```python
from build123d import *

# Parameters (mm, degrees)
SKETCH1_W           = 15
SKETCH1_H           = 45
BOSS_EXTRUDE1_DEPTH = 2.2
SKETCH1_3_W         = 20
SKETCH1_3_H         = 50
SKETCH1_3_W_2       = 15
SKETCH1_3_H_2       = 45
BOSS_EXTRUDE2_DEPTH = 2.5
SKETCH1_4_W         = 20
SKETCH1_4_H         = 50
SKETCH1_4_R         = 4.1
BOSS_EXTRUDE3_DEPTH = 2.5
FILLET1_R           = 2
SKETCH1_5_R         = 3.1
BOSS_EXTRUDE4_DEPTH = 2.5
FILLET2_R           = 10
CUT_EXTRUDE2_DEPTH  = 4
SKETCH3_OUTSIDE_W   = 41.892
SKETCH3_OUTSIDE_H   = 119.192
CUT_EXTRUDE3_DEPTH  = 74.159346635


with BuildPart() as part:
    # Sketch1 → Boss-Extrude1 (new body)
    with BuildSketch(Plane(origin=(0, 0, 0), x_dir=(1, 0, 0), z_dir=(0, 1, 0))):
        Rectangle(SKETCH1_W, SKETCH1_H)
        with BuildLine():
            ThreePointArc((-3.894544437, -4.023993492), (-5.599998379, 0.004260474), (-3.88841703, 4.029914763))
            Line((-3.88841703, 4.029914763), (-3.88841703, 8.505312122))
            ThreePointArc((-3.88841703, 8.505312122), (-3.870707724, 8.925763598), (-3.817705253, 9.343236712))
            Line((-3.817705253, 9.343236712), (-2.664584371, 16.126741161))
            ThreePointArc((-2.664584371, 16.126741161), (-2.610617779, 16.555799687), (-2.593926654, 16.987916591))
            ThreePointArc((-2.593926654, 16.987916591), (0, 19.6), (2.606045235, 17.000007028))
            ThreePointArc((2.606045235, 17.000007028), (2.623754541, 16.579555552), (2.676757012, 16.162082438))
            Line((2.676757012, 16.162082438), (3.829877895, 9.378577989))
            ThreePointArc((3.829877895, 9.378577989), (3.882880366, 8.961104875), (3.900589672, 8.540653399))
            Line((3.900589672, 8.540653399), (3.900589672, 4.018133922))
            ThreePointArc((3.900589672, 4.018133922), (5.157678846, 2.181364004), (5.6, 0))
            ThreePointArc((5.6, 0), (5.156037667, -2.185240393), (3.894544437, -4.023993492))
            Line((3.894544437, -4.023993492), (3.894544437, -8.540646372))
            ThreePointArc((3.894544437, -8.540646372), (3.876835131, -8.961097847), (3.82383266, -9.378570962))
            Line((3.82383266, -9.378570962), (2.670711777, -16.16207541))
            ThreePointArc((2.670711777, -16.16207541), (2.617709306, -16.579548524), (2.6, -17))
            ThreePointArc((2.6, -17), (0, -19.6), (-2.6, -17))
            ThreePointArc((-2.6, -17), (-2.617709306, -16.579548524), (-2.670711777, -16.16207541))
            Line((-2.670711777, -16.16207541), (-3.82383266, -9.378570962))
            ThreePointArc((-3.82383266, -9.378570962), (-3.876835131, -8.961097847), (-3.894544437, -8.540646372))
            Line((-3.894544437, -8.540646372), (-3.894544437, -4.023993492))
        make_face(mode=Mode.SUBTRACT)
    extrude(amount=-BOSS_EXTRUDE1_DEPTH)

    # Sketch1<3> → Boss-Extrude2 (add)
    # profile 1 of 2: a face of its own
    with BuildSketch(Plane(origin=(0, 0, 0), x_dir=(1, 0, 0), z_dir=(0, 1, 0))):
        Rectangle(SKETCH1_3_W, SKETCH1_3_H)
        Rectangle(SKETCH1_3_W_2, SKETCH1_3_H_2, mode=Mode.SUBTRACT)
    # profile 2 of 2: a face of its own
    with BuildSketch(Plane(origin=(0, 0, 0), x_dir=(1, 0, 0), z_dir=(0, 1, 0))):
        Rectangle(SKETCH1_3_W_2, SKETCH1_3_H_2)
        with BuildLine():
            ThreePointArc((-3.894544437, -4.023993492), (-5.599998379, 0.004260474), (-3.88841703, 4.029914763))
            Line((-3.88841703, 4.029914763), (-3.88841703, 8.505312122))
            ThreePointArc((-3.88841703, 8.505312122), (-3.870707724, 8.925763598), (-3.817705253, 9.343236712))
            Line((-3.817705253, 9.343236712), (-2.664584371, 16.126741161))
            ThreePointArc((-2.664584371, 16.126741161), (-2.610617779, 16.555799687), (-2.593926654, 16.987916591))
            ThreePointArc((-2.593926654, 16.987916591), (0, 19.6), (2.606045235, 17.000007028))
            ThreePointArc((2.606045235, 17.000007028), (2.623754541, 16.579555552), (2.676757012, 16.162082438))
            Line((2.676757012, 16.162082438), (3.829877895, 9.378577989))
            ThreePointArc((3.829877895, 9.378577989), (3.882880366, 8.961104875), (3.900589672, 8.540653399))
            Line((3.900589672, 8.540653399), (3.900589672, 4.018133922))
            ThreePointArc((3.900589672, 4.018133922), (5.157678846, 2.181364004), (5.6, 0))
            ThreePointArc((5.6, 0), (5.156037667, -2.185240393), (3.894544437, -4.023993492))
            Line((3.894544437, -4.023993492), (3.894544437, -8.540646372))
            ThreePointArc((3.894544437, -8.540646372), (3.876835131, -8.961097847), (3.82383266, -9.378570962))
            Line((3.82383266, -9.378570962), (2.670711777, -16.16207541))
            ThreePointArc((2.670711777, -16.16207541), (2.617709306, -16.579548524), (2.6, -17))
            ThreePointArc((2.6, -17), (0, -19.6), (-2.6, -17))
            ThreePointArc((-2.6, -17), (-2.617709306, -16.579548524), (-2.670711777, -16.16207541))
            Line((-2.670711777, -16.16207541), (-3.82383266, -9.378570962))
            ThreePointArc((-3.82383266, -9.378570962), (-3.876835131, -8.961097847), (-3.894544437, -8.540646372))
            Line((-3.894544437, -8.540646372), (-3.894544437, -4.023993492))
        make_face(mode=Mode.SUBTRACT)
    extrude(amount=-BOSS_EXTRUDE2_DEPTH)

    # Sketch1<4> → Boss-Extrude3 (add)
    with BuildSketch(Plane(origin=(0, 0, 0), x_dir=(1, 0, 0), z_dir=(0, 1, 0))):
        Rectangle(SKETCH1_4_W, SKETCH1_4_H)
        with Locations(Location((0, 0, 0), (0, 0, 270))):
            Circle(SKETCH1_4_R, mode=Mode.SUBTRACT)
    extrude(amount=BOSS_EXTRUDE3_DEPTH)

    # Fillet1
    fillet1_edges = [part.edges().sort_by_distance(p)[0] for p in [
        (-3.88841703, -1.25, -4.029914763),
        (-3.894544437, -1.25, 4.023993492),
        (3.894544437, -1.25, 4.023993492),
        (3.900589672, -1.25, -4.018133922),
    ]]
    fillet(fillet1_edges, radius=FILLET1_R)

    # Sketch1<5> → Boss-Extrude4 (add, symmetric)
    with BuildSketch(Plane(origin=(0, 0, 0), x_dir=(1, 0, 0), z_dir=(0, 1, 0))):
        with BuildLine():
            ThreePointArc((-10, 62.3), (0, 72.3), (10, 62.3))
            Line((10, 62.3), (10, 25))
            Line((10, 25), (-10, 25))
            Line((-10, 25), (-10, 62.3))
        make_face()
        with Locations(Location((0, 62.3, 0), (0, 0, 270))):
            Circle(SKETCH1_5_R, mode=Mode.SUBTRACT)
    extrude(amount=BOSS_EXTRUDE4_DEPTH, both=True)

    # Fillet2
    fillet2_edges = [part.edges().sort_by_distance(p)[0] for p in [
        (10, 0, 25),
        (-10, 0, 25),
    ]]
    fillet(fillet2_edges, radius=FILLET2_R - 0.0001)  # a hair under: the kernel refuses the full size

    # Sketch2 → Cut-Extrude2 (cut)
    # profile 1 of 4: a face of its own
    with BuildSketch(Plane.XZ.offset(2.5)):
        Polygon((5.973502692, -40.744870683), (-2.986751346, -35.571665602), (-2.986751346, -45.918075763), align=None)
        Polygon((5.773502692, -40.744870683), (-2.886751346, -35.744870683), (-2.886751346, -45.744870683), align=None, mode=Mode.SUBTRACT)
    # profile 2 of 4: a face of its own
    with BuildSketch(Plane.XZ.offset(2.5)):
        Polygon((5.973502692, -24.744870683), (-2.986751346, -19.571665602), (-2.986751346, -29.918075763), align=None)
        Polygon((5.773502692, -24.744870683), (-2.886751346, -19.744870683), (-2.886751346, -29.744870683), align=None, mode=Mode.SUBTRACT)
    # profile 3 of 4: a face of its own
    with BuildSketch(Plane.XZ.offset(2.5)):
        Polygon((-3.086751346, -48.744870683), (5.873502692, -43.571665602), (5.873502692, -53.918075763), align=None)
        Polygon((5.773502692, -53.744870683), (-2.886751346, -48.744870683), (5.773502692, -43.744870683), align=None, mode=Mode.SUBTRACT)
    # profile 4 of 4: a face of its own
    with BuildSketch(Plane.XZ.offset(2.5)):
        Polygon((-3.086751346, -32.744870683), (5.873502692, -27.571665602), (5.873502692, -37.918075763), align=None)
        Polygon((5.773502692, -37.744870683), (-2.886751346, -32.744870683), (5.773502692, -27.744870683), align=None, mode=Mode.SUBTRACT)
    extrude(amount=-CUT_EXTRUDE2_DEPTH, mode=Mode.SUBTRACT)

    # Sketch3 outside → Cut-Extrude3 (cut, through all)
    with BuildSketch(Plane.XZ.offset(2.5)):
        with Locations((0, -23.65)):
            Rectangle(SKETCH3_OUTSIDE_W, SKETCH3_OUTSIDE_H)
        with BuildLine():
            Line((10, -51.256214284), (10, 15))
            ThreePointArc((10, 15), (7.071067812, 22.071067812), (0, 25))
            ThreePointArc((0, 25), (-7.071067812, 22.071067812), (-10, 15))
            Line((-10, 15), (-10, -52.147572729))
            add(Edge.make_bspline(
                [(10, -51.256214284), (9.785135746, -51.909968828), (9.078957117, -53.953043182), (7.795150781, -57.091457155), (6.013003778, -60.33910848), (4.122796637, -62.728314915), (2.078800951, -64.258582197), (-0.15, -64.79554013), (-2.378800951, -64.258582197), (-4.422796637, -62.728314915), (-6.313003778, -60.33910848), (-8.095150781, -57.091457155), (-9.260115035, -54.243566479), (-9.877905488, -52.501784004), (-10, -52.147572729)],
                knots=[0.471097659, 0.471097659, 0.471097659, 0.471097659, 0.474472001, 0.481696232, 0.487703698, 0.492583405, 0.496543603, 0.5, 0.503456397, 0.507416595, 0.512296302, 0.518303768, 0.525527999, 0.527365119, 0.527365119, 0.527365119, 0.527365119], degree=3))
        make_face(mode=Mode.SUBTRACT)
    extrude(amount=-CUT_EXTRUDE3_DEPTH, mode=Mode.SUBTRACT)


solid = part.part
```
Could you check a few things on this model? Use its own coordinates, in mm. A direction names the side the tool comes from. Coordinates: 2 decimals unless noted, no trailing zeros. Order: outer loops, then holes, each group sorted by start corner. A loop starts at its lowest first (then second) coordinate and runs counter-clockwise, first axis right, second up. Notation, with made-up numbers: M 31,62.5 L 51,62.5 A25 cw 51,88.5 Z; hole C 37,-39.5 d5. An arc over 180 degrees is marked long. Use one line per item in the form item = value. Start each with the question number.
1. Suppose I cut it at C-C on z = 12.5. Write out the boundary of the cut face in (x, y).
2. On a 3-axis mill with a long thin cutter (end or side, diameter ignored), from which of +Z, -Z, +X, -X, +Y, -Y can I reach the whole of each face in a straight line? I mean faces 4 (the flat face through (1, -2.5, -41)), 5 (the cylindrical face through (5.6, -1.2, 0)). Say none if no direction works.
3. We'd pull the mould along Z, two halves only. Please class faces 1 (the flat face through (0, -2.5, -20)), 2 (the cylindrical face through (7.15, -0.04, 21.99)), 3 (the flat face through (3.901, -1, -7)): +Z half, -Z half, draft (parallel to the pull), parting line (faces both ways), or undercut.
4. For pin 1 (2 mm diameter, centred on x = -7.5, y = -1, fed in from -Z); pin 2 (2 mm diameter, centred on x = 0.5, y = 1, fed in from -Z), each with a flat end and sliding along its axis, tell me the tip position at first contact or that it passes through.
5. Suppose I cut it at A-A on z = 0. Write out the boundary of the cut face in (x, y), then the cut area to 3 significant figures.
6. Suppose I cut it at D-D on z = -29. Write out the boundary of the cut face in (x, y).
7. Suppose I cut it at B-B on y = -1.15. Count the separate pieces of the cut face and the enclosed holes in it, then the cut area to 3 significant figures.
8. Please list where these lines run through material, in increasing order: line 1 (X direction, y = -0.2, z = -7.5); line 2 (X direction, y = 1.35, z = 0); line 3 (Z direction, x = -1.5, y = 2.05).
Geometry says:
q1.outline = M -10,-2.5 L -3.29,-2.5 L -3.29,0 L 3.29,0 L 3.29,-2.5 L 10,-2.5 L 10,2.5 L -10,2.5 Z
q2.face_4 = +Z, -Z, +X, -X, -Y
q2.face_5 = -Y
q3.face_1 = draft
q3.face_2 = +Z half
q3.face_3 = undercut
q4.pin_1 = -59.88
q4.pin_2 = -59.59
q5.outline = M -10,-2.5 L -5.6,-2.5 L -5.6,0 L -4.1,0 L -4.1,2.5 L -10,2.5 Z; M 4.1,0 L 5.6,0 L 5.6,-2.5 L 10,-2.5 L 10,2.5 L 4.1,2.5 Z
q5.area = 51.5 mm^2
q6.outline = M -10,-2.5 L -2.99,-2.5 L -2.99,1.5 L -2.89,1.5 L -2.89,-2.5 L -1.6,-2.5 L -1.6,1.5 L -1.4,1.5 L -1.4,-2.5 L 3.4,-2.5 L 3.4,1.5 L 3.6,1.5 L 3.6,-2.5 L 5.77,-2.5 L 5.77,1.5 L 5.87,1.5 L 5.87,-2.5 L 10,-2.5 L 10,2.5 L -10,2.5 Z
q7.separate_pieces = 5
q7.enclosed_holes = 5
q7.area = 1,350 mm^2
q8.line_1 = -10 to -3.89, 3.9 to 10
q8.line_2 = -10 to -4.1, 4.1 to 10
q8.line_3 = -59.59 to -3.82, 3.82 to 24.89
